Can you work these out from the model? Positions are in its coordinate system, mm. A direction names the side the tool comes from. Give positions to 0.01 mm unless a question says otherwise; leave off trailing zeros. Order: outer loops, then holes, each group sorted by start corner. A loop starts at its lowest first (then second) coordinate and runs counter-clockwise, first axis right, second up. Notation, with made-up numbers: (24.25, 61.5) -> (72.25, 61.5) arc R33 ccw to (72.25, 100.5) -> close; hole circle Ø3 at (45, -25.75). An arc over 180 degrees is marked (long way). Answer as a JSON object with one key per item and string values.
```python
from build123d import *

# Parameters (mm, degrees)
SKETCH1_R                = 2.75
BOSS_EXTRUDE1_DEPTH      = 2
BOSS_EXTRUDE2_DEPTH      = 2.5
BOSS_EXTRUDE2_DEPTH_BACK = 0.5
FILLET1_R                = 3
CUT_EXTRUDE1_DEPTH       = 4.9
CUT_EXTRUDE1_DEPTH_BACK  = 3.5
FILLET2_R                = 3
SKETCH5_R                = 5.220153254
CUT_EXTRUDE2_DEPTH       = 3.5
SKETCH6_R                = 5.221148533
CUT_EXTRUDE3_DEPTH       = 3.5


with BuildPart() as part:
    # Sketch1 → Boss-Extrude1 (new body)
    with BuildSketch(Plane.XY):
        with BuildLine():
            Line((9.508808554, 0), (5, 0))
            ThreePointArc((5, 0), (1.464466094, -1.464466094), (0, -5))
            ThreePointArc((0, -5), (1.464466094, -8.535533906), (5, -10))
            Line((5, -10), (9.508808554, -10))
            ThreePointArc((9.508808554, -10), (9.996319776, -9.970105151), (10.476525698, -9.880868576))
            Line((10.476525698, -9.880868576), (19.242535625, -7.689366094))
            ThreePointArc((19.242535625, -7.689366094), (19.788205438, -7.334635803), (20, -6.719223594))
            Line((20, -6.719223594), (20, -4.609611797))
            Line((20, -4.609611797), (20, -3.280776406))
            ThreePointArc((20, -3.280776406), (19.788205438, -2.665364197), (19.242535625, -2.310633906))
            Line((19.242535625, -2.310633906), (10.476525698, -0.119131424))
            ThreePointArc((10.476525698, -0.119131424), (9.996319776, -0.029894849), (9.508808554, 0))
        make_face()
        with Locations((5, -5)):
            Circle(SKETCH1_R, mode=Mode.SUBTRACT)
    extrude(amount=BOSS_EXTRUDE1_DEPTH)

    # Sketch3 → Boss-Extrude2 (add, two sides: drawn at the far end of the back side and taken through both)
    with BuildSketch(Plane(origin=(0, -4, 0), x_dir=(-1, 0, 0), z_dir=(0, -1, 0)).offset(-BOSS_EXTRUDE2_DEPTH_BACK)):
        with BuildLine():
            ThreePointArc((-23.720153254, 5), (-23.109616483, 2.550217177), (-21.420820041, 0.673475957))
            Line((-21.420820041, 0.673475957), (-23.720153254, 5))
        make_face()
        with BuildLine():
            ThreePointArc((-21.420820041, 0.673475957), (-20.735912548, 0.282935757), (-20, 0))
            Line((-20, 0), (-20, 2.695113886))
            ThreePointArc((-20, 2.695113886), (-19.81101106, 7.417384951), (-15.75, 5))
            ThreePointArc((-15.75, 5), (-15.856067672, 4.243612637), (-16.166088613, 3.54557309))
            Line((-16.166088613, 3.54557309), (-14.069681773, 2.23915223))
            ThreePointArc((-14.069681773, 2.23915223), (-13.481188382, 3.564197108), (-13.279846746, 5))
            ThreePointArc((-13.279846746, 5), (-18.5, 10.220153254), (-23.720153254, 5))
            Line((-23.720153254, 5), (-21.420820041, 0.673475957))
        make_face()
        with BuildLine():
            Line((-20, 2.695113886), (-20, 0))
            ThreePointArc((-20, 0), (-16.65605263, 0.11636835), (-14.069681773, 2.23915223))
            Line((-14.069681773, 2.23915223), (-16.166088613, 3.54557309))
            ThreePointArc((-16.166088613, 3.54557309), (-17.904456328, 2.315260211), (-20, 2.695113886))
        make_face()
        with BuildLine():
            ThreePointArc((-13.279846746, 5), (-13.481188382, 3.564197108), (-14.069681773, 2.23915223))
            Line((-14.069681773, 2.23915223), (-10.476525698, 0))
            Line((-10.476525698, 0), (-13.279846746, 5))
        make_face()
        with BuildLine():
            ThreePointArc((-14.069681773, 2.23915223), (-16.65605263, 0.11636835), (-20, 0))
            ThreePointArc((-20, 0), (-20.735912548, 0.282935757), (-21.420820041, 0.673475957))
            Line((-21.420820041, 0.673475957), (-20, -2))
            Line((-20, -2), (-10.476525698, 0))
            Line((-10.476525698, 0), (-14.069681773, 2.23915223))
        make_face()
    extrude(amount=BOSS_EXTRUDE2_DEPTH + BOSS_EXTRUDE2_DEPTH_BACK)

    # Fillet1
    fillet1_edges = [part.edges().sort_by_distance(p)[0] for p in [
        (10.476525698, -5, 0),
        (21.420820041, -5, -0.673475957),
        (13.279846746, -5, -5),
    ]]
    fillet(fillet1_edges, radius=FILLET1_R)

    # Sketch4 → Cut-Extrude1 (cut, two sides: drawn at the far end of the back side and taken through both)
    with BuildSketch(Plane(origin=(0, -4, 0), x_dir=(-1, 0, 0), z_dir=(0, -1, 0)).offset(-CUT_EXTRUDE1_DEPTH_BACK)):
        Polygon((-21.432511864, 0.575653333), (-18.613235122, -2), (-20, -2), align=None)
    extrude(amount=CUT_EXTRUDE1_DEPTH + CUT_EXTRUDE1_DEPTH_BACK, mode=Mode.SUBTRACT)

    # Fillet2
    fillet2_edges = [part.edges().sort_by_distance(p)[0] for p in [
        (18.613235122, -5, 2),
    ]]
    fillet(fillet2_edges, radius=FILLET2_R)

    # Sketch5 → Cut-Extrude2 (cut)
    with BuildSketch(Plane.XZ.offset(6.5)):
        with Locations((18.5, -5)):
            Circle(SKETCH5_R)
    extrude(amount=CUT_EXTRUDE2_DEPTH, mode=Mode.SUBTRACT)

    # Sketch6 → Cut-Extrude3 (cut)
    with BuildSketch(Plane(origin=(0, -3.5, 0), x_dir=(1, 0, 0), z_dir=(0, 1, 0))):
        with Locations((18.5, 5)):
            Circle(SKETCH6_R)
    extrude(amount=CUT_EXTRUDE3_DEPTH, mode=Mode.SUBTRACT)


solid = part.part
```
1. Will these pins go through, and if not, where does the flat tip stop? pin 1 Ø3 at (x, y) = (8, -6.5) entering from -Z; pin 2 Ø4 at (x, y) = (4, -3.5) entering from -Z; pin 3 Ø5.5 at (x, z) = (17, -3) entering from +Y; pin 4 Ø6 at (x, z) = (3, -4) entering from +Y.
Worked answers:
{"pin 1": "z = -0.1", "pin 2": "z = 0", "pin 3": "y = -3.5", "pin 4": "through"}
2. For faces 1 (the face through (18.48, -2.83, 0.22)), 2 (the face through (10.25, -5.02, -0.42)), 3 (the face through (8, -5, 0)), which set-ups out of +Z, -Z, +X, -X, +Y, -Y let a thin tool reach every point of the face, with its end or its side?
Worked answers:
{"face 1": "-Z, +Y", "face 2": "-Z, -X, +Y, -Y", "face 3": "-Z, -X"}
3. If we section it at C-C on z = -6.25: Please give me the cut outline in (x, y).
Worked answers:
{"outline": "(13.43, -6.5) -> (16.05, -6.5) -> (16.05, -3.5) -> (13.43, -3.5) -> close; (20.95, -6.5) -> (23.57, -6.5) -> (23.57, -3.5) -> (20.95, -3.5) -> close"}
4. Please list where these lines run through material, in increasing order: L1, parallel to Y at x = 5, z = 0.6; L2, parallel to Z at x = 7.75, y = -3.5; L3, parallel to Y at x = 18.75, z = -1.25.
Worked answers:
{"L1": "-10 to -7.75, -2.25 to 0", "L2": "0 to 2", "L3": "-6.5 to -3.5"}
5. If we section it at A-A on x = 3: Please give me the cut outline in (y, z).
Worked answers:
{"outline": "(-9.58, 0) -> (-6.89, 0) -> (-6.89, 2) -> (-9.58, 2) -> close; (-3.11, 0) -> (-0.42, 0) -> (-0.42, 2) -> (-3.11, 2) -> close"}
6. If we mould it in two halves opening along X, with no side actions, what happens to faces 4 (the face through (12.13, -4.98, -2.95)), 5 (the face through (10, -0.03, 0.99)), 6 (the face through (9, -5, 2)), 7 (the face through (6.27, -7.44, 0.99))? For each: +X half, -X half, draft (parallel to the pull), parting line (faces both ways), or undercut.
Worked answers:
{"face 4": "-X half", "face 5": "+X half", "face 6": "draft", "face 7": "undercut"}
7. If we section it at B-B on y = -5.25: Please give me the cut outline in (x, z), then the cut area to 3 significant figures.
Worked answers:
{"outline": "(0.01, 0) -> (2.26, 0) -> (2.26, 2) -> (0.01, 2) -> close; (7.74, 0) -> (8.72, 0) arc R3 cw to (11.34, -1.53) -> (12.94, -4.4) arc R3 cw to (13.31, -5.55) arc R5.22 ccw (long way) to (21.84, -0.99) arc R3 cw to (21.43, -0.58) -> (19.47, 1.21) arc R3 ccw to (17.45, 2) -> (7.74, 2) -> close; hole circle Ø5.5 at (18.5, -5)", "area": "102 mm²"}
8. If we section it at D-D on x = 18.5: Please give me the cut outline in (y, z) (3 decimals), then the cut area to 3 significant figures.
Worked answers:
{"outline": "(-7.875, 0.22) -> (-6.5, 0.22) -> (-6.5, -2.25) -> (-3.5, -2.25) -> (-3.5, 0.221) -> (-2.125, 0.221) -> (-2.125, 1.81) -> (-7.875, 1.81) -> close; (-6.5, -10.22) -> (-3.5, -10.22) -> (-3.5, -7.75) -> (-6.5, -7.75) -> close", "area": "24.0 mm²"}
